from build123d import *

# Parameters (mm, degrees)
SKETCH1_W                    = 90
SKETCH1_H                    = 75
BOSS_EXTRUDE1_DEPTH          = 3
TAP_DRILL_FOR_M3X0_5_TAP1_D  = 2.5
FILLET1_R                    = 3
CSK_FOR_M3_SFHCS1_AT_2_COUNT = 2
CSK_FOR_M3_SFHCS1_AT_2_PITCH = 31.5
CSK_FOR_M3_SFHCS1_AT_3_COUNT = 2
CSK_FOR_M3_SFHCS1_AT_3_PITCH = 85.97819491
CSK_FOR_M3_SFHCS1_AT_4_COUNT = 2
CSK_FOR_M3_SFHCS1_AT_4_PITCH = 80


with BuildPart() as part:
    # Sketch1 → Boss-Extrude1 (new body)
    with BuildSketch(Plane(origin=(0, 0, 0), x_dir=(1, 0, 0), z_dir=(0, 1, 0))):
        Rectangle(SKETCH1_W, SKETCH1_H)
    extrude(amount=BOSS_EXTRUDE1_DEPTH)

    # Tap Drill for M3x0.5 Tap1 (through all)
    with Locations(Plane(origin=(0, 3, 0), x_dir=(1, 0, 0), z_dir=(0, 1, 0))):
        with Locations((-41, 33.5), (-41, -33.5), (41, -33.5), (41, 33.5)):
            Hole(TAP_DRILL_FOR_M3X0_5_TAP1_D / 2)

    # Fillet1
    fillet1_edges = [part.edges().sort_by_distance(p)[0] for p in [
        (-45, 1.5, -37.5),
        (45, 1.5, -37.5),
        (45, 1.5, 37.5),
        (-45, 1.5, 37.5),
    ]]
    fillet(fillet1_edges, radius=FILLET1_R)

    # Sketch7 → CSK for M3 SFHCS1 (revolve, cut)
    with BuildSketch(Plane(origin=(-40, 3, -7), x_dir=(0, 0, 1), z_dir=(1, 0, 0))):
        Polygon((0, 0), (0, 3), (1.6, 3), (1.6, 1.76), (3.36, 0), align=None)
    csk_for_m3_sfhcs1 = revolve(axis=Axis((-40, 9.35, -7), (0, -1, 0)), mode=Mode.SUBTRACT)

    # CSK for M3 SFHCS1 at 2: CSK for M3 SFHCS1 ×2
    with Locations(*[(0, 0, i * CSK_FOR_M3_SFHCS1_AT_2_PITCH) for i in range(1, CSK_FOR_M3_SFHCS1_AT_2_COUNT)]):
        add(csk_for_m3_sfhcs1, mode=Mode.SUBTRACT)

    # CSK for M3 SFHCS1 at 3: CSK for M3 SFHCS1 ×2
    with Locations(*[Vector(0.9304684761484525, 0, 0.36637196248345316) * (i * CSK_FOR_M3_SFHCS1_AT_3_PITCH) for i in range(1, CSK_FOR_M3_SFHCS1_AT_3_COUNT)]):
        add(csk_for_m3_sfhcs1, mode=Mode.SUBTRACT)

    # CSK for M3 SFHCS1 at 4: CSK for M3 SFHCS1 ×2
    with Locations(*[(i * CSK_FOR_M3_SFHCS1_AT_4_PITCH, 0, 0) for i in range(1, CSK_FOR_M3_SFHCS1_AT_4_COUNT)]):
        add(csk_for_m3_sfhcs1, mode=Mode.SUBTRACT)


solid = part.part
Part model, mm, in its own coordinate system. Give positions to 0.01 mm unless a question says otherwise; leave off trailing zeros. Order: outer loops, then holes, each group sorted by start corner. A loop starts at its lowest first (then second) coordinate and runs counter-clockwise, first axis right, second up. Notation, with made-up numbers: (38, 80) - (49, 80) arc R18 cw to (49, 108) - close; hole circle Ø2 at (64, 72.25). An arc over 180 degrees is marked (long way). One line per question, with ' | ' between items.
1. Band-saw the part on B-B on y = 2.2. Give the number of separate pieces and of enclosed holes in the cut face, then the cut area to 3 significant figures.
Filled in:
separate pieces: 1 | enclosed holes: 8 | area: 6,640 mm²
2. Drill centre lines: probe 1 along X at (y, z) = (0.6, 24.5); probe 2 along X at (y, z) = (1.4, 33.5); probe 3 along Z at (x, y) = (-41, 0.8). Where is each one in solid material? Low to high.
Filled in:
probe 1: -45 to -41.6, -38.4 to 38.4, 41.6 to 45 | probe 2: -45 to -42.25, -39.75 to 39.75, 42.25 to 45 | probe 3: -37.5 to -34.75, -32.25 to -8.25, -5.75 to 23.25, 25.75 to 32.25, 34.75 to 37.5
3. Drop flat-ended pins along their axis: P1, Ø3.5, axis at x = 40, z = -7, coming from the +Y side; P2, Ø1.5, axis at x = -41, z = 33.5, coming from the -Y side. Give the stop position or say it passes through.
Filled in:
P1: y = 1.39 | P2: through
4. Band-saw the part on C-C on z = 33.5. List the corners of the cut face in (x, y).
Filled in:
outline: (-45, 0) - (-42.25, 0) - (-42.25, 3) - (-45, 3) - close; (-39.75, 0) - (39.75, 0) - (39.75, 3) - (-39.75, 3) - close; (42.25, 0) - (45, 0) - (45, 3) - (42.25, 3) - close
5. Pull direction Z, two halves, no side cores. Call faces 1 (the face through (41.42, 0.63, -6.26)), 2 (the face through (-38.58, 0.63, -6.26)), 3 (the face through (-44.14, 1.52, -36.6)), 4 (the face through (-44.14, 1.52, 36.6)): +Z half, -Z half, draft (parallel to the pull), parting line (faces both ways), or undercut.
Filled in:
face 1: undercut | face 2: undercut | face 3: -Z half | face 4: +Z half
6. Band-saw the part on A-A on z = -7. List the corners of the cut face in (x, y), then the cut area to 3 significant figures.
Filled in:
outline: (-45, 0) - (-41.6, 0) - (-41.6, 1.24) - (-43.36, 3) - (-45, 3) - close; (-38.4, 0) - (38.4, 0) - (38.4, 1.24) - (36.64, 3) - (-36.64, 3) - (-38.4, 1.24) - close; (41.6, 0) - (45, 0) - (45, 3) - (43.36, 3) - (41.6, 1.24) - close | area: 245 mm²
